from build123d import *

# Parameters (mm, degrees)
SKETCH17_W                   = 46
SKETCH17_H                   = 26
BASE_FLANGE4_DEPTH           = 1
EDGE_FLANGE1_STRIP_W         = 5.4732
EDGE_FLANGE1_STRIP_H         = 1
EDGE_FLANGE1_STRIP_CUT_DEPTH = 26
EDGE_FLANGE1_DEPTH           = 26
SKETCH30_W                   = 26
SKETCH30_H                   = 22
TAB1_DEPTH                   = 1
SKETCHED_BEND3_DEPTH         = 26
SKETCHED_START               = 22
SKETCHED_BEND3_2_DEPTH       = 4
SKETCHED_BEND3_3_DEPTH       = 26
SKETCHED_BEND3_4_DEPTH       = 22
EDGE_FLANGE2_STRIP_W         = 5.4732
EDGE_FLANGE2_STRIP_H         = 1
EDGE_FLANGE2_STRIP_CUT_DEPTH = 25.028776631
EDGE_FLANGE2_DEPTH           = 25.028776631
EDGE_FLANGE3_STRIP_W         = 5.4732
EDGE_FLANGE3_STRIP_H         = 1
EDGE_FLANGE3_STRIP_CUT_DEPTH = 26
EDGE_FLANGE3_DEPTH           = 26
SKETCH40_W                   = 26
SKETCH40_H                   = 22
TAB2_DEPTH                   = 1
SKETCHED_BEND4_DEPTH         = 26
SKETCHED_BEND4_2_DEPTH       = 4
SKETCHED_BEND4_3_DEPTH       = 22
SKETCHED_BEND4_4_DEPTH       = 4
EDGE_FLANGE4_STRIP_W         = 5.4732
EDGE_FLANGE4_STRIP_H         = 1
EDGE_FLANGE4_STRIP_CUT_DEPTH = 25.028776631
EDGE_FLANGE4_DEPTH           = 25.028776631
SKETCH47_R                   = 5
CUT_EXTRUDE1_DEPTH           = 10


# Read off the part's stored shape, not the designer's step: Sketched Bend3, Sketched Bend4
# Sheet-metal steps are written as plain solids
with BuildPart() as part:
    # Sketch17 → Base-Flange4 (new body)
    with BuildSketch(Plane.XY):
        with Locations((23, 13)):
            Rectangle(SKETCH17_W, SKETCH17_H)
    extrude(amount=-BASE_FLANGE4_DEPTH)

    # Edge-Flange1 strip (across the edge) → Edge-Flange1 strip cut (cut)
    with BuildSketch(Plane(origin=(46, 0, 0), x_dir=(-1, 0, 0), z_dir=(0, 1, 0))):
        with Locations((-1, -0.5)):
            Rectangle(EDGE_FLANGE1_STRIP_W, EDGE_FLANGE1_STRIP_H)
    extrude(amount=EDGE_FLANGE1_STRIP_CUT_DEPTH, mode=Mode.SUBTRACT)

    # Edge-Flange1 section (across the edge) → Edge-Flange1 (add)
    with BuildSketch(Plane(origin=(46, 0, 0), x_dir=(-1, 0, 0), z_dir=(0, 1, 0))):
        with BuildLine():
            Line((0, 0.7366), (0, 14))
            Line((0, 14), (1, 14))
            Line((1, 14), (1, 0.7366))
            ThreePointArc((1, 0.7366), (1.215745145, 0.215745145), (1.7366, 0))
            Line((1.7366, 0), (1.7366, -1))
            ThreePointArc((1.7366, -1), (0.508638364, -0.491361636), (0, 0.7366))
        make_face()
    extrude(amount=EDGE_FLANGE1_DEPTH)

    # Sketch30 → Tab1 (add)
    with BuildSketch(Plane(origin=(46, 0, 0), x_dir=(0, 0, -1), z_dir=(1, 0, 0))):
        with Locations((-27, 11)):
            Rectangle(SKETCH30_W, SKETCH30_H)
    extrude(amount=-TAB1_DEPTH)

    # Sketched Bend3 outline → Sketched Bend3 (cut)
    with BuildSketch(Plane(origin=(0, 0, 0), x_dir=(1, 0, 0), z_dir=(0, 1, 0))):
        with BuildLine():
            Line((46, -13.398582279), (46, -0.7366))
            ThreePointArc((46, -0.7366), (45.491361636, 0.491361636), (44.2634, 1))
            Line((44.2634, 1), (0, 1))
            Line((0, 1), (0, 0))
            Line((0, 0), (44.2634, 0))
            ThreePointArc((44.2634, 0), (44.784254855, -0.215745145), (45, -0.7366))
            Line((45, -0.7366), (45, -14.971223369))
            ThreePointArc((45, -14.971223369), (45.271171885, -14.039397205), (46, -13.398582279))
        make_face()
    extrude(amount=SKETCHED_BEND3_DEPTH, mode=Mode.SUBTRACT)

    # Sketched Bend3 2 outline → Sketched Bend3 2 (cut)
    with BuildSketch(Plane(origin=(0, 0, 0), x_dir=(1, 0, 0), z_dir=(0, 1, 0)).offset(SKETCHED_START)):
        with BuildLine():
            Line((45.296980354, -14), (45.765376631, -14))
            Line((45.765376631, -14), (45.508638364, -13.743261733))
            ThreePointArc((45.508638364, -13.743261733), (45.396646229, -13.866549911), (45.296980354, -14))
        make_face()
    extrude(amount=SKETCHED_BEND3_2_DEPTH, mode=Mode.SUBTRACT)

    # Sketched Bend3 3 outline → Sketched Bend3 3 (add)
    with BuildSketch(Plane(origin=(0, 0, 0), x_dir=(1, 0, 0), z_dir=(0, 1, 0))):
        with BuildLine():
            Line((46.7366, -14.234623369), (59.028776631, -14.234623369))
            ThreePointArc((59.028776631, -14.234623369), (60.256738267, -13.725985005), (60.765376631, -12.498023369))
            Line((60.765376631, -12.498023369), (60.765376631, 31.765376631))
            Line((60.765376631, 31.765376631), (59.765376631, 31.765376631))
            Line((59.765376631, 31.765376631), (59.765376631, -12.498023369))
            ThreePointArc((59.765376631, -12.498023369), (59.549631486, -13.018878224), (59.028776631, -13.234623369))
            Line((59.028776631, -13.234623369), (46.7366, -13.234623369))
            ThreePointArc((46.7366, -13.234623369), (46.359286442, -13.276108612), (46, -13.398582279))
            Line((46, -13.398582279), (46, -14))
            Line((46, -14), (45.765376631, -14))
            Line((45.765376631, -14), (46.215745145, -14.450368514))
            ThreePointArc((46.215745145, -14.450368514), (46.454715384, -14.290693705), (46.7366, -14.234623369))
        make_face()
    extrude(amount=SKETCHED_BEND3_3_DEPTH)

    # Sketched Bend3 4 outline → Sketched Bend3 4 (add)
    with BuildSketch(Plane(origin=(0, 0, 0), x_dir=(1, 0, 0), z_dir=(0, 1, 0))):
        with BuildLine():
            ThreePointArc((46, -14.971223369), (46.056070336, -14.689338753), (46.215745145, -14.450368514))
            Line((46.215745145, -14.450368514), (46, -14.234623369))
            Line((46, -14.234623369), (46, -14.971223369))
        make_face()
    extrude(amount=SKETCHED_BEND3_4_DEPTH)

    # Edge-Flange2 strip (across the edge) → Edge-Flange2 strip cut (cut)
    with BuildSketch(Plane(origin=(45, 22, 40), x_dir=(0, -1, 0), z_dir=(0, 0, -1))):
        with Locations((-1, -0.5)):
            Rectangle(EDGE_FLANGE2_STRIP_W, EDGE_FLANGE2_STRIP_H)
    extrude(amount=EDGE_FLANGE2_STRIP_CUT_DEPTH, mode=Mode.SUBTRACT)

    # Edge-Flange2 section (across the edge) → Edge-Flange2 (add)
    with BuildSketch(Plane(origin=(45, 22, 40), x_dir=(0, -1, 0), z_dir=(0, 0, -1))):
        with BuildLine():
            Line((0, 0.7366), (0, 5))
            Line((0, 5), (1, 5))
            Line((1, 5), (1, 0.7366))
            ThreePointArc((1, 0.7366), (1.215745145, 0.215745145), (1.7366, 0))
            Line((1.7366, 0), (1.7366, -1))
            ThreePointArc((1.7366, -1), (0.508638364, -0.491361636), (0, 0.7366))
        make_face()
    extrude(amount=EDGE_FLANGE2_DEPTH)

    # Edge-Flange3 strip (across the edge) → Edge-Flange3 strip cut (cut)
    with BuildSketch(Plane(origin=(59.765376631, 26, -31.765376631), x_dir=(0, 0, 1), z_dir=(0, -1, 0))):
        with Locations((-1, -0.5)):
            Rectangle(EDGE_FLANGE3_STRIP_W, EDGE_FLANGE3_STRIP_H)
    extrude(amount=EDGE_FLANGE3_STRIP_CUT_DEPTH, mode=Mode.SUBTRACT)

    # Edge-Flange3 section (across the edge) → Edge-Flange3 (add)
    with BuildSketch(Plane(origin=(59.765376631, 26, -31.765376631), x_dir=(0, 0, 1), z_dir=(0, -1, 0))):
        with BuildLine():
            Line((0, 0.7366), (0, 14))
            Line((0, 14), (1, 14))
            Line((1, 14), (1, 0.7366))
            ThreePointArc((1, 0.7366), (1.215745145, 0.215745145), (1.7366, 0))
            Line((1.7366, 0), (1.7366, -1))
            ThreePointArc((1.7366, -1), (0.508638364, -0.491361636), (0, 0.7366))
        make_face()
    extrude(amount=EDGE_FLANGE3_DEPTH)

    # Sketch40 → Tab2 (add)
    with BuildSketch(Plane(origin=(0, 0, -31.765376631), x_dir=(-1, 0, 0), z_dir=(0, 0, -1))):
        with Locations((-32.765376631, 11)):
            Rectangle(SKETCH40_W, SKETCH40_H)
    extrude(amount=-TAB2_DEPTH)

    # Sketched Bend4 outline → Sketched Bend4 (cut)
    with BuildSketch(Plane(origin=(0, 0, 0), x_dir=(1, 0, 0), z_dir=(0, 1, 0))):
        with BuildLine():
            Line((45.16395891, 31.765376631), (19.765376631, 31.765376631))
            Line((19.765376631, 31.765376631), (19.765376631, 30.765376631))
            Line((19.765376631, 30.765376631), (46.7366, 30.765376631))
            ThreePointArc((46.7366, 30.765376631), (45.804773836, 31.036548516), (45.16395891, 31.765376631))
        make_face()
    extrude(amount=SKETCHED_BEND4_DEPTH, mode=Mode.SUBTRACT)

    # Sketched Bend4 2 outline → Sketched Bend4 2 (cut)
    with BuildSketch(Plane(origin=(0, 0, 0), x_dir=(1, 0, 0), z_dir=(0, 1, 0)).offset(SKETCHED_START)):
        Polygon((45.765376631, 31.530753262), (46, 31.765376631), (45.765376631, 31.765376631), align=None)
    extrude(amount=SKETCHED_BEND4_2_DEPTH, mode=Mode.SUBTRACT)

    # Sketched Bend4 3 outline → Sketched Bend4 3 (add)
    with BuildSketch(Plane(origin=(0, 0, 0), x_dir=(1, 0, 0), z_dir=(0, 1, 0))):
        with BuildLine():
            Line((46, 32.501976631), (46, 57.530753262))
            Line((46, 57.530753262), (45, 57.530753262))
            Line((45, 57.530753262), (45, 32.501976631))
            ThreePointArc((45, 32.501976631), (45.041485243, 32.124663073), (45.16395891, 31.765376631))
            Line((45.16395891, 31.765376631), (46.7366, 31.765376631))
            ThreePointArc((46.7366, 31.765376631), (46.215745145, 31.981121776), (46, 32.501976631))
        make_face()
    extrude(amount=SKETCHED_BEND4_3_DEPTH)

    # Sketched Bend4 4 outline → Sketched Bend4 4 (add)
    with BuildSketch(Plane(origin=(0, 0, 0), x_dir=(1, 0, 0), z_dir=(0, 1, 0)).offset(SKETCHED_START)):
        with BuildLine():
            ThreePointArc((46.7366, 31.765376631), (46.454715384, 31.821446967), (46.215745145, 31.981121776))
            Line((46.215745145, 31.981121776), (46, 31.765376631))
            Line((46, 31.765376631), (46.7366, 31.765376631))
        make_face()
        with BuildLine():
            Line((45.765376631, 31.062356985), (45.765376631, 31.530753262))
            Line((45.765376631, 31.530753262), (45.508638364, 31.274014995))
            ThreePointArc((45.508638364, 31.274014995), (45.631926542, 31.16202286), (45.765376631, 31.062356985))
        make_face()
    extrude(amount=SKETCHED_BEND4_4_DEPTH)

    # Edge-Flange4 strip (across the edge) → Edge-Flange4 strip cut (cut)
    with BuildSketch(Plane(origin=(45, 22, -32.501976631), x_dir=(0, -1, 0), z_dir=(0, 0, -1))):
        with Locations((-1, -0.5)):
            Rectangle(EDGE_FLANGE4_STRIP_W, EDGE_FLANGE4_STRIP_H)
    extrude(amount=EDGE_FLANGE4_STRIP_CUT_DEPTH, mode=Mode.SUBTRACT)

    # Edge-Flange4 section (across the edge) → Edge-Flange4 (add)
    with BuildSketch(Plane(origin=(45, 22, -32.501976631), x_dir=(0, -1, 0), z_dir=(0, 0, -1))):
        with BuildLine():
            Line((0, 0.7366), (0, 5))
            Line((0, 5), (1, 5))
            Line((1, 5), (1, 0.7366))
            ThreePointArc((1, 0.7366), (1.215745145, 0.215745145), (1.7366, 0))
            Line((1.7366, 0), (1.7366, -1))
            ThreePointArc((1.7366, -1), (0.508638364, -0.491361636), (0, 0.7366))
        make_face()
    extrude(amount=EDGE_FLANGE4_DEPTH)

    # Sketch47 → Cut-Extrude1 (cut)
    with BuildSketch(Plane(origin=(60.765376631, 0, 0), x_dir=(0, 0, -1), z_dir=(1, 0, 0))):
        with Locations((8.765376631, 13)):
            Circle(SKETCH47_R)
    extrude(amount=-CUT_EXTRUDE1_DEPTH, mode=Mode.SUBTRACT)


solid = part.part
Input: part model. Units: mm. Frame: model coordinates. A direction names the side the tool comes from. Coordinates: 2 decimals unless noted, no trailing zeros. Order: outer loops, then holes, each group sorted by start corner. A loop starts at its lowest first (then second) coordinate and runs counter-clockwise, first axis right, second up. Notation, with made-up numbers: M 79,-33.75 L 138,-33.75 A25 ccw 138,-15.75 Z; hole C -37.5,46 d9. An arc over 180 degrees is marked long. Answer as CSV lines item,"result".
1. Pull-direction query (Z, two-part tool) for faces 1 (the flat face through (53, 13, -30.765)), 2 (the cylindrical face through (60.24, 12.82, 13.74)), 3 (the flat face through (45, 10, 28)); classes: released by +Z, released by -Z, zero draft, split by the parting line, or undercut.
Reported:
face 1,"undercut"
face 2,"released by +Z"
face 3,"zero draft"
2. Section A-A (y = 13). Return the cut outline in (x, z).
Reported:
outline,"M 45,-57.53 L 46,-57.53 L 46,-32.5 A0.74 cw 46.74,-31.77 L 59.03,-31.77 A1.74 ccw 60.77,-30.03 L 60.77,-13.77 L 59.77,-13.77 L 59.77,-30.03 A0.74 cw 59.03,-30.77 L 46.74,-30.77 A1.74 ccw 45,-32.5 Z; M 45,14.97 A1.74 ccw 46.74,13.23 L 59.03,13.23 A0.74 cw 59.77,12.5 L 59.77,-3.77 L 60.77,-3.77 L 60.77,12.5 A1.74 ccw 59.03,14.23 L 46.74,14.23 A0.74 cw 46,14.97 L 46,40 L 45,40 Z"
3. Section C-C (z = -5). Return the cut outline in (x, y).
Reported:
outline,"M 59.77,0 L 60.77,0 L 60.77,9.71 L 59.77,9.71 Z; M 59.77,16.29 L 60.77,16.29 L 60.77,26 L 59.77,26 Z"
4. Section B-B (x = 55.5). Return the cut outline in (y, z), then the cut area to 3 significant figures.
Reported:
outline,"M 0,-31.77 L 26,-31.77 L 26,-30.77 L 0,-30.77 Z; M 0,13.23 L 26,13.23 L 26,14.23 L 0,14.23 Z"
area,"52.0 mm2"
5. Section D-D (y = 3.5). Return the cut outline in (x, z), then the cut area to 3 significant figures.
Reported:
outline,"M 45,-57.53 L 46,-57.53 L 46,-32.5 A0.74 cw 46.74,-31.77 L 59.03,-31.77 A1.74 ccw 60.77,-30.03 L 60.77,12.5 A1.74 ccw 59.03,14.23 L 46.74,14.23 A0.74 cw 46,14.97 L 46,40 L 45,40 L 45,14.97 A1.74 ccw 46.74,13.23 L 59.03,13.23 A0.74 cw 59.77,12.5 L 59.77,-30.03 A0.74 cw 59.03,-30.77 L 46.74,-30.77 A1.74 ccw 45,-32.5 Z"
area,"125 mm2"
6. First-contact query: P1, Ø10, axis at y = 13, z = -40.5, coming from the -X side; P2, Ø3.5, axis at x = 51.5, y = 11.5, coming from the +Z side; P3, Ø3.5, axis at x = 43, z = 22, coming from the +Y side; P4, Ø1.5, axis at y = 23, z = -44, coming from the -X side. Flat tips, straight axial feed; report the tip coordinate or a pass-through.
Reported:
P1,"x = 45"
P2,"z = 14.23"
P3,"y = 22"
P4,"through"
7. Material intervals for line 1 (Z direction, x = 51.75, y = 2); line 2 (X direction, y = 16.75, z = -14.5); line 3 (X direction, y = 2.5, z = 30.5), sorted ascending. Write a range as from..to.
Reported:
line 1,"-31.77..-30.77, 13.23..14.23"
line 2,"59.77..60.77"
line 3,"45..46"
8. Access query for faces 4 (the flat face through (53, 13, -31.765)), 5 (the flat face through (53, 13, 13.235)), 6 (the cylindrical face through (45.5, 21.48, 27.66)), 7 (the flat face through (42, 21, 28)). Directions: +Z, -Z, +X, -X, +Y, -Y. A direction counts if a zero-diameter tool reaches every point of the face in a straight line with its end or side. Return the directions, or none.
Reported:
face 4,"-Z, +X, +Y, -Y"
face 5,"-X, +Y, -Y"
face 6,"+Z, +X, +Y"
face 7,"+Z, -Z, -X, -Y"
